The model under review builds one solid part; all positions refer to its coordinate system, in mm. Face numbers are marked on the shaded views. A direction names the side the tool comes from. Round coordinates to 2 decimals unless told otherwise and drop trailing zeros. Write each loop counter-clockwise with the first axis right and the second up, starting at its lowest first coordinate (ties: lowest second). Pieces come first, ordered by that corner, then holes.
Item 1: Add section A-A (x = 31.5). Give the boundary of the cut face in (y, z).
Item 2: Add section D-D (y = 3.25). Give the boundary of the cut face in (x, z), plus the area to 3 significant figures.
Item 3: Machinability: for the marked faces 1, 2 and 3, which of the approach directions +Z, -Z, +X, -X, +Y, -Y give a long, thin tool a straight path to every point of the face, cutting with its end or side? Answer none if there is none.
Item 4: To check wall thickness, follow L1, parallel to X at y = 0.6, z = -5 (3 decimals); L2, parallel to Y at x = 22, z = -3; L3, parallel to X at y = 3.5, z = -8. State the ranges of each line that lie inside material, in increasing order.
Item 5: Clearance check with flat-ended pins moving along their axes: pin 1 Ø1.2 at (y, z) = (6, -4.5) entering from +X (3 decimals); pin 2 Ø3.5 at (x, z) = (25.655, -5) entering from -Y. State where each tip first meets the part, or that it passes through.
Item 6: Add section B-B (y = 8). Give the boundary of the cut face in (x, z), plus the area to 3 significant figures.
Item 7: Draft analysis for pull direction Z (two halves, no side actions). For the marked faces 4, 5 and 6, state which applies: +Z half, -Z half, draft (parallel to the pull), parting line (faces both ways), or undercut.
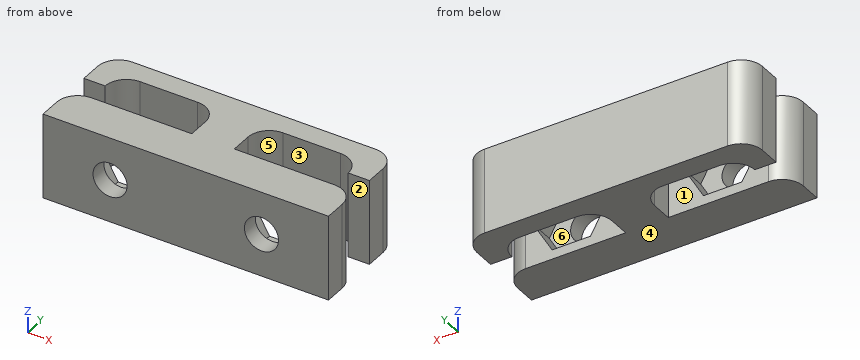
```python
from build123d import *

# Parameters (mm, degrees)
SKETCH2_W           = 33.53
SKETCH2_H           = 10
SKETCH2_R           = 2
BOSS_EXTRUDE1_DEPTH = 5
CUT_EXTRUDE1_DEPTH  = 3
BOSS_EXTRUDE2_DEPTH = 10
FILLET1_START       = -11
FILLET1_DEPTH       = 12
FILLET1_START_2     = -10
FILLET1_2_DEPTH     = 10


with BuildPart() as part:
    # Sketch2 → Boss-Extrude1 (new body)
    with BuildSketch(Plane(origin=(0, 0, 0), x_dir=(1, 0, 0), z_dir=(0, 1, 0))):
        with Locations((16.765, 5)):
            Rectangle(SKETCH2_W, SKETCH2_H)
        with Locations(Location((7.875, 5, 0), (0, 0, 270))):
            Circle(SKETCH2_R, mode=Mode.SUBTRACT)
        with Locations(Location((25.655, 5, 0), (0, 0, 270))):
            Circle(SKETCH2_R, mode=Mode.SUBTRACT)
    extrude(amount=BOSS_EXTRUDE1_DEPTH)

    # Sketch3 → Cut-Extrude1 (cut)
    with BuildSketch(Plane(origin=(0, 5, 0), x_dir=(1, 0, 0), z_dir=(0, 1, 0))):
        Polygon((12.3783321, 5), (10.12666605, 8.9), (5.62333395, 8.9), (3.3716679, 5), (5.62333395, 1.1), (10.12666605, 1.1), align=None)
        Polygon((30.1583321, 5), (27.90666605, 8.9), (23.40333395, 8.9), (21.1516679, 5), (23.40333395, 1.1), (27.90666605, 1.1), align=None)
    extrude(amount=-CUT_EXTRUDE1_DEPTH, mode=Mode.SUBTRACT)

    # Sketch4 → Boss-Extrude2 (add)
    with BuildSketch(Plane(origin=(0, 0, -10), x_dir=(-1, 0, 0), z_dir=(0, 0, -1))):
        Polygon((-14.265, 5), (-14.265, 10), (-2.5, 10), (-2.5, 7.5), (0, 7.5), (0, 12.5), (-33.53, 12.5), (-33.53, 7.5), (-31.03, 7.5), (-31.03, 10), (-19.265, 10), (-19.265, 5), align=None)
    extrude(amount=-BOSS_EXTRUDE2_DEPTH)

    # Fillet1: read off the stored shape, not the designer's step
    # Fillet1 outline → Fillet1 (cut)
    with BuildSketch(Plane.XY.offset(FILLET1_START)):
        with BuildLine():
            Line((33.53, 12.5), (31.03, 12.5))
            ThreePointArc((31.03, 12.5), (32.797766953, 11.767766953), (33.53, 10))
            Line((33.53, 10), (33.53, 12.5))
        make_face()
        with BuildLine():
            ThreePointArc((0, 10), (0.732233047, 11.767766953), (2.5, 12.5))
            Line((2.5, 12.5), (0, 12.5))
            Line((0, 12.5), (0, 10))
        make_face()
        with BuildLine():
            Line((33.53, 5), (31.03, 5))
            ThreePointArc((31.03, 5), (32.797766953, 4.267766953), (33.53, 2.5))
            Line((33.53, 2.5), (33.53, 5))
        make_face()
        with BuildLine():
            ThreePointArc((0, 2.5), (0.732233047, 4.267766953), (2.5, 5))
            Line((2.5, 5), (0, 5))
            Line((0, 5), (0, 2.5))
        make_face()
    extrude(amount=FILLET1_DEPTH, mode=Mode.SUBTRACT)

    # Fillet1 2 outline → Fillet1 2 (add)
    with BuildSketch(Plane.XY.offset(FILLET1_START_2)):
        with BuildLine():
            Line((31.03, 10), (28.53, 10))
            ThreePointArc((28.53, 10), (30.297766953, 9.267766953), (31.03, 7.5))
            Line((31.03, 7.5), (31.03, 10))
        make_face()
        with BuildLine():
            Line((19.265, 10), (19.265, 7.5))
            ThreePointArc((19.265, 7.5), (19.997233047, 9.267766953), (21.765, 10))
            Line((21.765, 10), (19.265, 10))
        make_face()
        with BuildLine():
            ThreePointArc((2.5, 7.5), (3.232233047, 9.267766953), (5, 10))
            Line((5, 10), (2.5, 10))
            Line((2.5, 10), (2.5, 7.5))
        make_face()
        with BuildLine():
            ThreePointArc((11.765, 10), (13.532766953, 9.267766953), (14.265, 7.5))
            Line((14.265, 7.5), (14.265, 10))
            Line((14.265, 10), (11.765, 10))
        make_face()
    extrude(amount=FILLET1_2_DEPTH)


solid = part.part
```
Numbers:
1. outline: (0, -10) - (4.96, -10) - (4.96, 0) - (0, 0) - close; (7.5, -10) - (12.46, -10) - (12.46, 0) - (7.5, 0) - close
2. outline: (0.12, -10) - (33.41, -10) - (33.41, 0) - (0.12, 0) - close; hole (3.37, -5) - (5.62, -8.9) - (10.13, -8.9) - (12.38, -5) - (10.13, -1.1) - (5.62, -1.1) - close; hole (21.15, -5) - (23.4, -8.9) - (27.91, -8.9) - (30.16, -5) - (27.91, -1.1) - (23.4, -1.1) - close
2. area: 228 mm2
3. face 1: +Z, -Z, -X
3. face 2: +Z, -Z, +X
3. face 3: +Z, -Z
4. L1: x = 0 to 5.875, 9.875 to 23.655, 27.655 to 33.53
4. L2: y = 0 to 5, 10 to 12.5
4. L3: x = 0.21 to 5.1, 10.65 to 22.88, 28.43 to 33.32
5. pin 1: stops at x = 19.265
5. pin 2: stops at y = 10
6. outline: (0, -10) - (2.55, -10) - (2.55, 0) - (0, 0) - close; (14.21, -10) - (19.32, -10) - (19.32, 0) - (14.21, 0) - close; (30.98, -10) - (33.53, -10) - (33.53, 0) - (30.98, 0) - close
6. area: 102 mm2
7. face 4: -Z half
7. face 5: draft
7. face 6: undercut
